```python
from build123d import *

# Parameters (mm, degrees)
F0_R     = 9.5191370384
F1_DEPTH = 3.175
F2_R     = 9.5191370384
F3_DEPTH = 6.35


with BuildPart() as f1:
    # F0 (on Top) → F1 (new body)
    with BuildSketch(Plane.XY):
        Circle(F0_R)
        with BuildLine():
            ThreePointArc((0, 8.6135921563), (6.0907294241, 6.0907294241), (8.6135921563, 0))
            ThreePointArc((8.6135921563, 0), (6.0907294241, -6.0907294241), (0, -8.6135921563))
            ThreePointArc((0, -8.6135921563), (-8.6135921563, 0), (0, 8.6135921563))
        make_face(mode=Mode.SUBTRACT)
        with BuildLine():
            ThreePointArc((0, -8.6135921563), (6.0907294241, -6.0907294241), (8.6135921563, 0))
            ThreePointArc((8.6135921563, 0), (6.0907294241, 6.0907294241), (0, 8.6135921563))
            Line((0, 8.6135921563), (0, -8.6135921563))
        make_face()
    extrude(amount=F1_DEPTH)

    # F2 (on face) → F3 (join)
    with BuildSketch(Plane.XY.offset(3.175)):
        Circle(F2_R)
        with BuildLine():
            ThreePointArc((0, 8.6092061915), (6.0876280786, 6.0876280786), (8.6092061915, 0))
            ThreePointArc((8.6092061915, 0), (6.0876280786, -6.0876280786), (0, -8.6092061915))
            Line((0, -8.6092061915), (0, -8.6135921563))
            ThreePointArc((0, -8.6135921563), (-8.6135921563, 0), (0, 8.6135921563))
            Line((0, 8.6135921563), (0, 8.6092061915))
        make_face(mode=Mode.SUBTRACT)
    extrude(amount=F3_DEPTH)


solid = f1.part
```
Source: CAD feature listing. Evaluate the final solid. Frame: model axes, mm. A direction names the side the tool comes from. Round coordinates to 2 decimals unless told otherwise and drop trailing zeros. Loops run counter-clockwise (first coordinate to the right, second up) from the corner with the lowest first, then second, coordinate; pieces in that order, holes last. Notation, with made-up numbers: M -3,-26.5 L 32,-26.5 A23 cw 32,10.5 Z; hole C 8,30.25 d5. An arc over 180 degrees is marked long. Use a Markdown table: item, result. Add a question column.
1. Section query B-B on x = -0.5. Return the cut outline in (y, z) (3 decimals).
2. Reachability of faces 4 (the flat face through (3, 0, 3.175)), 5 (the flat face through (-9, -1, 9.525)) from +Z, -Z, +X, -X, +Y, -Y: full face, straight path, thin tool, end or side. Return the list, or none.
3. Section query D-D on y = -6. Return the cut outline in (x, z) (3 decimals), then the cut area to 3 significant figures.
4. Line query: line 1 (Y direction, x = 0, z = 6); line 2 (Z direction, x = 7.5, y = 1) (3 decimals); line 3 (Y direction, x = 2.5, z = 6). Output: solid intervals per line, ascending.
5. Mould query, pull axis Y, two halves, no side actions, for faces 1 (the cylindrical face through (-8.61, -0.19, 4.7)), 2 (the cylindrical face through (-7.554, -5.792, 4.696)), 3 (the flat face through (2, 0, 0)). Classes: pulls with the +Y half, pulls with the -Y half, needs draft (parallel to the pull), parting line crosses it, or undercut.
6. Contact query for flat-ended pins moving along their axis: P1, Ø4, axis at x = 3.5, z = 4.5, coming from the -Y side; P2, Ø2.5, axis at x = 4.5, y = 4, coming from the +Z side (3 decimals); P3, Ø1, axis at x = 3, z = 1, coming from the -Y side (3 decimals); P4, Ø3, axis at x = -5.5, y = -3, coming from the +Z side. Output: stop coordinate, or through.
7. Section query A-A on y = -3.5. Return the cut outline in (x, z) (3 decimals), then the cut area to 3 significant figures.
Reported:
| question | item | result |
|---|---|---|
| 1 | outline | M -9.506,0 L -8.599,0 L -8.599,9.525 L -9.506,9.525 Z; M 8.599,0 L 9.506,0 L 9.506,9.525 L 8.599,9.525 Z |
| 2 | face 4 | +Z |
| 2 | face 5 | +Z, +X, -X, +Y, -Y |
| 3 | outline | M -7.39,0 L -6.18,0 L -6.18,9.525 L -7.39,9.525 Z; M 0,0 L 7.39,0 L 7.39,9.525 L 6.174,9.525 L 6.174,3.175 L 0,3.175 Z |
| 3 | area | 42.7 mm² |
| 4 | line 1 | y = -9.52 to -8.61, 8.61 to 9.52 |
| 4 | line 2 | z = 0 to 3.175 |
| 4 | line 3 | y = -9.18 to -8.24, 8.24 to 9.18 |
| 5 | face 1 | undercut |
| 5 | face 2 | parting line crosses it |
| 5 | face 3 | needs draft |
| 6 | P1 | stops at y = -9.4 |
| 6 | P2 | stops at z = 3.175 |
| 6 | P3 | stops at y = -9.185 |
| 6 | P4 | passes through |
| 7 | outline | M -8.852,0 L -7.87,0 L -7.87,9.525 L -8.852,9.525 Z; M 0,0 L 8.852,0 L 8.852,9.525 L 7.866,9.525 L 7.866,3.175 L 0,3.175 Z |
| 7 | area | 43.7 mm² |
